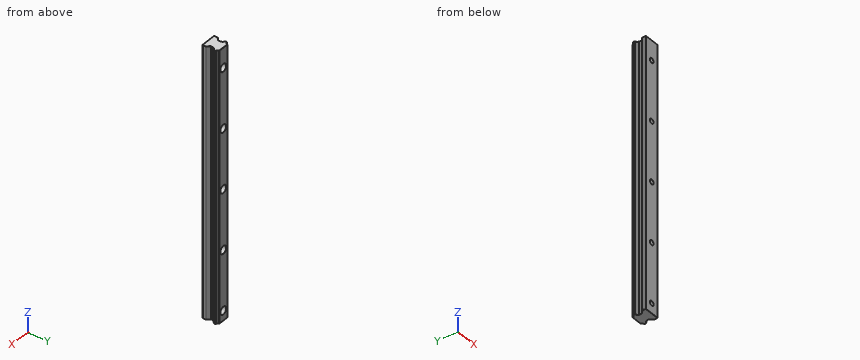
```python
from build123d import *

# Parameters (mm, degrees)
BODY_DEPTH                                 = 270
AESTHETIC_CHAMFER_SIZE                     = 0.15
PRODUCTION_FILLET_R                        = 0.1
MOUNTING_HOLES_PATTERN_COUNT               = 5
MOUNTING_HOLES_PATTERN_PITCH               = 60
PRODUCTION_FILLET_OF_MOUNTING_HOLES_PATT_R = 0.1


with BuildPart() as part:
    # Rail Profile → Body (new body)
    with BuildSketch(Plane.XY):
        with BuildLine():
            Line((-7, 0), (7, 0))
            Line((7, 0), (7.5, 0.5))
            Line((7.5, 0.5), (7.5, 3.085786438))
            ThreePointArc((7.5, 3.085786438), (7.423879533, 3.46846987), (7.207106781, 3.792893219))
            Line((7.207106781, 3.792893219), (4.867157288, 6.132842712))
            ThreePointArc((4.867157288, 6.132842712), (4.780448187, 6.262612052), (4.75, 6.415685425))
            Line((4.75, 6.415685425), (4.75, 8.584314575))
            ThreePointArc((4.75, 8.584314575), (4.780448187, 8.737387948), (4.867157288, 8.867157288))
            Line((4.867157288, 8.867157288), (5.062965362, 9.062965362))
            ThreePointArc((5.062965362, 9.062965362), (5.134996734, 9.161242682), (5.17409812, 9.27664646))
            ThreePointArc((5.17409812, 9.27664646), (5.61862915, 10.13137085), (6.47335354, 10.57590188))
            ThreePointArc((6.47335354, 10.57590188), (6.694124352, 10.694306692), (6.801170165, 10.920803148))
            ThreePointArc((6.801170165, 10.920803148), (6.915305692, 11.154571658), (7.149074202, 11.268707185))
            ThreePointArc((7.149074202, 11.268707185), (7.399691242, 11.400760606), (7.5, 11.665685425))
            Line((7.5, 11.665685425), (7.5, 12.334314575))
            ThreePointArc((7.5, 12.334314575), (7.399691242, 12.599239394), (7.149074202, 12.731292815))
            ThreePointArc((7.149074202, 12.731292815), (6.915305692, 12.845428342), (6.801170165, 13.079196852))
            ThreePointArc((6.801170165, 13.079196852), (6.694124352, 13.305693308), (6.47335354, 13.42409812))
            ThreePointArc((6.47335354, 13.42409812), (5.61862915, 13.86862915), (5.17409812, 14.72335354))
            ThreePointArc((5.17409812, 14.72335354), (5.134996734, 14.838757318), (5.062965362, 14.937034638))
            Line((5.062965362, 14.937034638), (5, 15))
            Line((5, 15), (-5, 15))
            Line((-5, 15), (-5.062965362, 14.937034638))
            ThreePointArc((-5.062965362, 14.937034638), (-5.134996734, 14.838757318), (-5.17409812, 14.72335354))
            ThreePointArc((-5.17409812, 14.72335354), (-5.61862915, 13.86862915), (-6.47335354, 13.42409812))
            ThreePointArc((-6.47335354, 13.42409812), (-6.694124352, 13.305693308), (-6.801170165, 13.079196852))
            ThreePointArc((-6.801170165, 13.079196852), (-6.915305692, 12.845428342), (-7.149074202, 12.731292815))
            ThreePointArc((-7.149074202, 12.731292815), (-7.399691242, 12.599239394), (-7.5, 12.334314575))
            Line((-7.5, 12.334314575), (-7.5, 11.665685425))
            ThreePointArc((-7.5, 11.665685425), (-7.399691242, 11.400760606), (-7.149074202, 11.268707185))
            ThreePointArc((-7.149074202, 11.268707185), (-6.915305692, 11.154571658), (-6.801170165, 10.920803148))
            ThreePointArc((-6.801170165, 10.920803148), (-6.694124352, 10.694306692), (-6.47335354, 10.57590188))
            ThreePointArc((-6.47335354, 10.57590188), (-5.61862915, 10.13137085), (-5.17409812, 9.27664646))
            ThreePointArc((-5.17409812, 9.27664646), (-5.134996734, 9.161242682), (-5.062965362, 9.062965362))
            Line((-5.062965362, 9.062965362), (-4.867157288, 8.867157288))
            ThreePointArc((-4.867157288, 8.867157288), (-4.780448187, 8.737387948), (-4.75, 8.584314575))
            Line((-4.75, 8.584314575), (-4.75, 6.415685425))
            ThreePointArc((-4.75, 6.415685425), (-4.780448187, 6.262612052), (-4.867157288, 6.132842712))
            Line((-4.867157288, 6.132842712), (-7.207106781, 3.792893219))
            ThreePointArc((-7.207106781, 3.792893219), (-7.423879533, 3.46846987), (-7.5, 3.085786438))
            Line((-7.5, 3.085786438), (-7.5, 0.5))
            Line((-7.5, 0.5), (-7, 0))
        make_face()
    extrude(amount=-BODY_DEPTH)

    # Aesthetic Chamfer
    aesthetic_chamfer_edges = [part.edges().sort_by_distance(p)[0] for p in [
        (7.423879533, 3.46846987, -270),
        (-5.134996734, 9.161242682, -270),
        (-4.965061325, 8.965061325, -270),
        (-4.780448187, 8.737387948, -270),
        (-4.75, 7.5, -270),
        (-4.780448187, 6.262612052, -270),
        (-6.037132034, 4.962867966, -270),
        (-7.423879533, 3.46846987, -270),
        (-7.5, 1.792893219, -270),
        (-7.25, 0.25, -270),
        (0, 0, -270),
        (6.037132034, 4.962867966, -270),
        (4.780448187, 6.262612052, -270),
        (4.75, 7.5, -270),
        (4.780448187, 8.737387948, -270),
        (4.965061325, 8.965061325, -270),
        (5.134996734, 9.161242682, -270),
        (5.61862915, 10.13137085, -270),
        (6.694124352, 10.694306692, -270),
        (0, 0, 0),
        (-7.25, 0.25, 0),
        (-7.5, 1.792893219, 0),
        (-7.423879533, 3.46846987, 0),
        (-6.037132034, 4.962867966, 0),
        (-4.780448187, 6.262612052, 0),
        (6.915305692, 11.154571658, -270),
        (-4.75, 7.5, 0),
        (-4.780448187, 8.737387948, 0),
        (-4.965061325, 8.965061325, 0),
        (-5.134996734, 9.161242682, 0),
        (-5.61862915, 10.13137085, 0),
        (-6.694124352, 10.694306692, 0),
        (-6.915305692, 11.154571658, 0),
        (7.25, 0.25, -270),
        (7.399691242, 11.400760606, -270),
        (-7.399691242, 11.400760606, 0),
        (-7.5, 12, 0),
        (-7.399691242, 12.599239394, 0),
        (-6.915305692, 12.845428342, 0),
        (-6.694124352, 13.305693308, 0),
        (-5.61862915, 13.86862915, 0),
        (-5.134996734, 14.838757318, 0),
        (-5.031482681, 14.968517319, 0),
        (7.5, 12, -270),
        (0, 15, 0),
        (5.031482681, 14.968517319, 0),
        (5.134996734, 14.838757318, 0),
        (5.61862915, 13.86862915, 0),
        (6.694124352, 13.305693308, 0),
        (6.915305692, 12.845428342, 0),
        (7.399691242, 12.599239394, 0),
        (7.399691242, 12.599239394, -270),
        (7.5, 12, 0),
        (7.399691242, 11.400760606, 0),
        (6.915305692, 11.154571658, 0),
        (6.694124352, 10.694306692, 0),
        (5.61862915, 10.13137085, 0),
        (5.134996734, 9.161242682, 0),
        (4.965061325, 8.965061325, 0),
        (4.780448187, 8.737387948, 0),
        (6.915305692, 12.845428342, -270),
        (4.75, 7.5, 0),
        (4.780448187, 6.262612052, 0),
        (6.037132034, 4.962867966, 0),
        (7.423879533, 3.46846987, 0),
        (7.5, 1.792893219, 0),
        (7.25, 0.25, 0),
        (6.694124352, 13.305693308, -270),
        (5.61862915, 13.86862915, -270),
        (5.134996734, 14.838757318, -270),
        (5.031482681, 14.968517319, -270),
        (0, 15, -270),
        (-5.031482681, 14.968517319, -270),
        (7.5, 1.792893219, -270),
        (-5.134996734, 14.838757318, -270),
        (-5.61862915, 13.86862915, -270),
        (-6.694124352, 13.305693308, -270),
        (-6.915305692, 12.845428342, -270),
        (-7.399691242, 12.599239394, -270),
        (-7.5, 12, -270),
        (-7.399691242, 11.400760606, -270),
        (-6.915305692, 11.154571658, -270),
        (-6.694124352, 10.694306692, -270),
        (-5.61862915, 10.13137085, -270),
    ]]
    chamfer(aesthetic_chamfer_edges, length=AESTHETIC_CHAMFER_SIZE)

    # Sketch1 → Mounting Hole (revolve, cut)
    with BuildSketch(Plane(origin=(0, 15, -20), x_dir=(0, 0, 1), z_dir=(1, 0, 0))):
        Polygon((0, 0), (0, 15), (2.35, 15), (2.25, 14.9), (2.25, 5.4), (2.35, 5.3), (3.75, 5.3), (3.75, 0.1), (3.85, 0), align=None)
    mounting_hole = revolve(axis=Axis((0, 21.35, -20), (0, -1, 0)), mode=Mode.SUBTRACT)

    # Production Fillet
    production_fillet_edges = [part.edges().sort_by_distance(p)[0] for p in [
        (0, 9.7, -23.75),
    ]]
    fillet(production_fillet_edges, radius=PRODUCTION_FILLET_R)

    # Mounting Holes Pattern: Mounting Hole ×5
    with Locations(*[(0, 0, -i * MOUNTING_HOLES_PATTERN_PITCH) for i in range(1, MOUNTING_HOLES_PATTERN_COUNT)]):
        add(mounting_hole, mode=Mode.SUBTRACT)

    # Production Fillet of Mounting Holes Patt
    production_fillet_of_mounting_holes_patt_edges = [part.edges().sort_by_distance(p)[0] for p in [
        (0, 9.7, -83.75),
        (0, 9.7, -143.75),
        (0, 9.7, -203.75),
        (0, 9.7, -263.75),
    ]]
    fillet(production_fillet_of_mounting_holes_patt_edges, radius=PRODUCTION_FILLET_OF_MOUNTING_HOLES_PATT_R)


solid = part.part
```
For this review, take the finished solid that the model builds, in its own axes (mm). Round coordinates to 2 decimals unless told otherwise and drop trailing zeros. One line per question, with ' | ' between items. Start each with the question number.
1) Add section A-A (x = 0). Count the separate pieces of the cut face and the enclosed holes in it, and give its area (3 significant figures).
2) Wall thickness on line 1 along Z through (x, y) = (0, 6.5); line 2 along Z through (x, y) = (0, 11.3); line 3 along X through (y, z) = (7, -20): over which ranges is each line inside the solid? List them lowest first.
3) For pin 1 Ø3.5 at (x, z) = (0, -140) entering from -Y; pin 2 Ø6 at (x, z) = (0, -20) entering from +Y; pin 3 Ø1.1 at (y, z) = (8, -156) entering from +X, all flat-tipped, find the tip position at first contact; note any pin that passes through.
Reported:
1) separate pieces: 6 | enclosed holes: 0 | area: 3,630 mm²
2) line 1: z = -270 to -262.25, -257.75 to -202.25, -197.75 to -142.25, -137.75 to -82.25, -77.75 to -22.25, -17.75 to 0 | line 2: z = -270 to -263.75, -256.25 to -203.75, -196.25 to -143.75, -136.25 to -83.75, -76.25 to -23.75, -16.25 to 0 | line 3: x = -4.75 to -2.25, 2.25 to 4.75
3) pin 1: passes through | pin 2: stops at y = 9.7 | pin 3: stops at x = 4.75
